Source: CAD feature listing. Evaluate the final solid. Frame: model axes, mm. A direction names the side the tool comes from. Round coordinates to 2 decimals unless told otherwise and drop trailing zeros. Order: outer loops, then holes, each group sorted by start corner. A loop starts at its lowest first (then second) coordinate and runs counter-clockwise, first axis right, second up. Notation, with made-up numbers: (50.5, 21.5) -> (104.5, 21.5) arc R16 cw to (104.5, 36.5) -> close; hole circle Ø10 at (41, -5). An arc over 180 degrees is marked (long way). Write item = value, one per line. Start each with the question number.
(1) Draft query along X for faces 1 (the face through (23.46, 108.35, -3.99)), 2 (the face through (8, 111.291, -10)), 3 (the face through (24.129, 123.122, -3.986)), 4 (the face through (-13.632, 118.145, -3.986)). Return one class per face: released by +X, released by -X, zero draft, split by the parting line, or undercut.
(2) Cut plane A-A on z = -10.25. Return the cut outline in (x, y).
(3) Cut plane B-B on z = -20.75. Return the cut outline in (x, y).
(4) Reachability of faces 5 (the face through (26.31, 113.34, -5.7)), 6 (the face through (18.231, 120.763, -3.986)), 7 (the face through (26.487, 103.466, -3.986)) from +Z, -Z, +X, -X, +Y, -Y: full face, straight path, thin tool, end or side. Return the list, or none.
(5) Ray query, line 1 (Z direction, x = 19, y = 113); line 2 (Z direction, x = 14.5, y = 101.75); line 3 (X direction, y = 105.5, z = -10.75). Return the intervals inside material, ascending.
(6) Cut plane C-C on z = -14. Return the cut outline in (x, y).
(7) Contact query for flat-ended pins moving along their axis: pin 1 Ø12 at (x, z) = (5, -11) entering from -Y; pin 2 Ø6.5 at (x, y) = (-9.54, 118.29) entering from -Z; pin 3 Ø1.8 at (x, z) = (7.5, -8.5) entering from +Y; pin 4 Ø3.5 at (x, y) = (-9.54, 98.29) entering from -Z. Output: stop coordinate, or through.
from build123d import *

# Parameters (mm, degrees)
SKETCH1_R           = 2
BOSS_EXTRUDE1_DEPTH = 3
FILLET1_R           = 1
SKETCH2_W           = 6
SKETCH2_H           = 6
BOSS_EXTRUDE2_DEPTH = 13
FILLET4_R           = 1


with BuildPart() as part:
    # Sketch1 → Boss-Extrude1 (new body)
    with BuildSketch(Plane(origin=(0, 0, -3), x_dir=(-1, 0, 0), z_dir=(0, 0, -1))):
        with BuildLine():
            Line((-22.078522838, 93.957303237), (-14.489191473, 97.629560349))
            ThreePointArc((-14.489191473, 97.629560349), (-7.955777551, 99.127171578), (-1.42236363, 97.629560349))
            Line((-1.42236363, 97.629560349), (6.166967735, 93.957303237))
            ThreePointArc((6.166967735, 93.957303237), (8.247667355, 93.459042522), (10.346147194, 93.876124065))
            ThreePointArc((10.346147194, 93.876124065), (10.86613185, 94.129321852), (11.363439854, 94.424580911))
            ThreePointArc((11.363439854, 94.424580911), (13.629470969, 98.370815693), (11.75890266, 102.519145498))
            Line((11.75890266, 102.519145498), (9.424652508, 104.386545619))
            ThreePointArc((9.424652508, 104.386545619), (7.548127746, 108.290889666), (9.424652508, 112.195233714))
            Line((9.424652508, 112.195233714), (11.75890266, 114.062633835))
            ThreePointArc((11.75890266, 114.062633835), (13.629470969, 118.21096364), (11.363439854, 122.157198422))
            ThreePointArc((11.363439854, 122.157198422), (10.86613185, 122.452457481), (10.346147194, 122.705655268))
            ThreePointArc((10.346147194, 122.705655268), (8.247667355, 123.122736811), (6.166967735, 122.624476095))
            Line((6.166967735, 122.624476095), (-1.42236363, 118.952218983))
            ThreePointArc((-1.42236363, 118.952218983), (-7.955777551, 117.454607754), (-14.489191473, 118.952218983))
            Line((-14.489191473, 118.952218983), (-22.078522838, 122.624476095))
            ThreePointArc((-22.078522838, 122.624476095), (-24.159222457, 123.122736811), (-26.257702296, 122.705655268))
            ThreePointArc((-26.257702296, 122.705655268), (-26.777686952, 122.452457481), (-27.274994956, 122.157198422))
            ThreePointArc((-27.274994956, 122.157198422), (-29.541026071, 118.21096364), (-27.670457762, 114.062633835))
            Line((-27.670457762, 114.062633835), (-25.33620761, 112.195233714))
            ThreePointArc((-25.33620761, 112.195233714), (-23.459682848, 108.290889666), (-25.33620761, 104.386545619))
            Line((-25.33620761, 104.386545619), (-27.670457762, 102.519145498))
            ThreePointArc((-27.670457762, 102.519145498), (-29.541026071, 98.370815693), (-27.274994956, 94.424580911))
            ThreePointArc((-27.274994956, 94.424580911), (-26.777686952, 94.129321852), (-26.257702296, 93.876124065))
            ThreePointArc((-26.257702296, 93.876124065), (-24.159222457, 93.459042522), (-22.078522838, 93.957303237))
        make_face()
        with Locations((-25.455777551, 118.290889666)):
            Circle(SKETCH1_R, mode=Mode.SUBTRACT)
        with Locations((9.544222449, 118.290889666)):
            Circle(SKETCH1_R, mode=Mode.SUBTRACT)
        with Locations((-25.455777551, 98.290889666)):
            Circle(SKETCH1_R, mode=Mode.SUBTRACT)
        with Locations((9.544222449, 98.290889666)):
            Circle(SKETCH1_R, mode=Mode.SUBTRACT)
    extrude(amount=BOSS_EXTRUDE1_DEPTH)

    # Fillet1
    fillet1_edges = [part.edges().sort_by_distance(p)[0] for p in [
        (29.541026071, 98.370815693, -6),
        (26.777686952, 94.129321852, -6),
        (24.159222457, 93.459042522, -6),
        (18.283857155, 95.793431793, -6),
        (7.955777551, 99.127171578, -6),
        (-2.372302053, 95.793431793, -6),
        (-8.247667355, 93.459042522, -6),
        (-10.86613185, 94.129321852, -6),
        (-13.629470969, 98.370815693, -6),
        (-10.591777584, 103.452845558, -6),
        (23.459682848, 108.290889666, -6),
        (-7.548127746, 108.290889666, -6),
        (-10.591777584, 113.128933774, -6),
        (-13.629470969, 118.21096364, -6),
        (-10.86613185, 122.452457481, -6),
        (-8.247667355, 123.122736811, -6),
        (-2.372302053, 120.788347539, -6),
        (7.955777551, 117.454607754, -6),
        (18.283857155, 120.788347539, -6),
        (24.159222457, 123.122736811, -6),
        (26.777686952, 122.452457481, -6),
        (26.503332686, 103.452845558, -6),
        (29.541026071, 118.21096364, -6),
        (26.503332686, 113.128933774, -6),
    ]]
    fillet(fillet1_edges, radius=FILLET1_R)

    # Sketch2 → Boss-Extrude2 (add)
    with BuildSketch(Plane(origin=(0, 0, -6), x_dir=(-1, 0, 0), z_dir=(0, 0, -1))):
        with Locations((-7.955777551, 108.290889666)):
            Rectangle(SKETCH2_W, SKETCH2_H)
    extrude(amount=BOSS_EXTRUDE2_DEPTH)

    # Fillet4
    fillet4_edges = [part.edges().sort_by_distance(p)[0] for p in [
        (10.955777551, 108.290889666, -6),
        (7.955777551, 105.290889666, -6),
        (4.955777551, 108.290889666, -6),
        (7.955777551, 111.290889666, -6),
    ]]
    fillet(fillet4_edges, radius=FILLET4_R)

    # Sketch4 → Revolve2 (revolve)
    with BuildSketch(Plane(origin=(0, 108.290889666, 0), x_dir=(0, 0, -1), z_dir=(0, 1, 0))):
        with BuildLine():
            Line((12, -7.955777551), (32, -7.955777551))
            ThreePointArc((32, -7.955777551), (22, -17.955777551), (12, -7.955777551))
        make_face()
    revolve(axis=Axis((7.955777551, 108.290889666, -12), (0, 0, -1)))


solid = part.part
Evaluation:
q1.face_1 = released by +X
q1.face_2 = zero draft
q1.face_3 = undercut
q1.face_4 = released by -X
q2.outline = (4.96, 105.29) -> (10.96, 105.29) -> (10.96, 111.29) -> (4.96, 111.29) -> close
q3.outline = circle Ø19.84 at (7.96, 108.29)
q4.face_5 = -Z, +X
q4.face_6 = +Z, -Z, +Y
q4.face_7 = +Z, -Z, +X
q5.line_1 = -6 to -3
q5.line_2 = -25.79 to -18.21, -6 to -3
q5.line_3 = 4.96 to 10.96
q6.outline = circle Ø12 at (7.96, 108.29)
q7.pin_1 = 98.27
q7.pin_2 = -6
q7.pin_3 = 111.29
q7.pin_4 = through
